Verification items for this drawing (mm, ordinates from the low corner). A direction names the side the tool comes from. Coordinates: 2 decimals unless noted, no trailing zeros. Write each loop counter-clockwise with the first axis right and the second up, starting at its lowest first coordinate (ties: lowest second). Pieces come first, ordered by that corner, then holes. Notation, with made-up numbers: (53.25, 40) -> (76.25, 40) arc R25 cw to (76.25, 59) -> close; hole circle Ø7 at (-33, 4.25). An arc over 180 degrees is marked (long way). Answer as CSV lines item,"result".
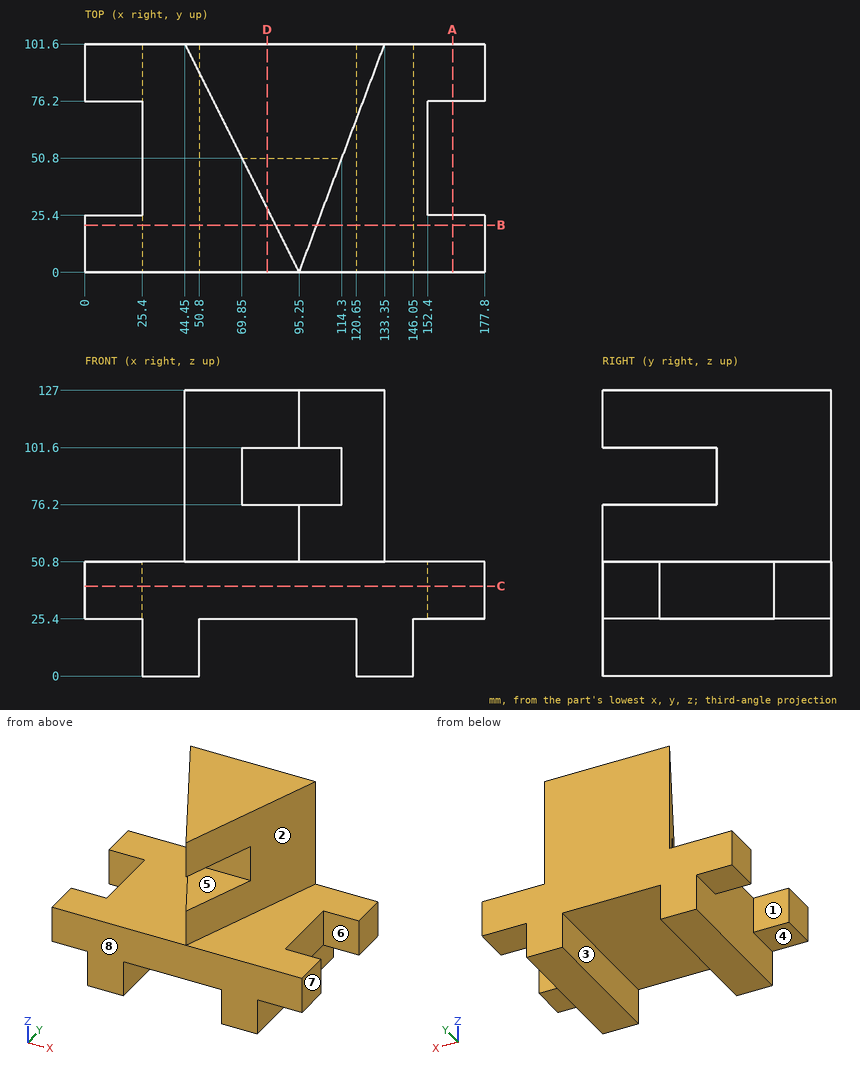
Item 1: Release check for a two-part mould opening along Y. For the marked faces 6, 7 and 8 record: +Y half, -Y half, draft (parallel to the pull), parting line (faces both ways), or undercut.
Responses:
face 6,"undercut"
face 7,"draft"
face 8,"-Y half"
Item 2: Cross-section at D-D, the plane x = 81. Record the cut outline in (y, z).
Responses:
outline,"(0, 25.4) -> (101.6, 25.4) -> (101.6, 127) -> (28.5, 127) -> (28.5, 101.6) -> (50.8, 101.6) -> (50.8, 76.2) -> (28.5, 76.2) -> (28.5, 50.8) -> (0, 50.8) -> close"
Item 3: Set-up check for the marked faces 1, 2, 3, 4 and 5: record each of +Z, -Z, +X, -X, +Y, -Y from which the full face is reachable in a straight line by a thin tool's end or side.
Responses:
face 1,"+Z, -Z, -X"
face 2,"+Z, +X, -Y"
face 3,"-Z, +Y, -Y"
face 4,"-Z, -X, +Y, -Y"
face 5,"+X, -X, -Y"
Item 4: Thickness scan on probe 1 along X at (y, z) = (32, 22); probe 2 along Z at (x, y) = (78, 89); probe 3 along Z at (x, y) = (152, 82.5). Record the ranges inside material, lowest first.
Responses:
probe 1,"x = 25.4 to 50.8, 120.65 to 146.05"
probe 2,"z = 25.4 to 127"
probe 3,"z = 25.4 to 50.8"
Item 5: Depth check by flat-ended pin: pin 1 Ø15 at (y, z) = (38, 22.5) entering from -X; pin 2 Ø4 at (x, y) = (91, 30.5) entering from -Z; pin 3 Ø1 at (x, y) = (53, 52.5) entering from +Z. Enter the tip coordinate at first touch or a pass-through.
Responses:
pin 1,"stops at x = 25.4"
pin 2,"stops at z = 25.4"
pin 3,"stops at z = 50.8"
Item 6: Cross-section at B-B, the plane y = 21. Record the cut outline in (x, z) (3 decimals).
Responses:
outline,"(0, 25.4) -> (25.4, 25.4) -> (25.4, 0) -> (50.8, 0) -> (50.8, 25.4) -> (120.65, 25.4) -> (120.65, 0) -> (146.05, 0) -> (146.05, 25.4) -> (177.8, 25.4) -> (177.8, 50.8) -> (103.125, 50.8) -> (103.125, 76.2) -> (84.75, 76.2) -> (84.75, 50.8) -> (0, 50.8) -> close; (84.75, 101.6) -> (103.125, 101.6) -> (103.125, 127) -> (84.75, 127) -> close"
Item 7: Cross-section at C-C, the plane z = 40. Record the cut outline in (x, y).
Responses:
outline,"(0, 0) -> (177.8, 0) -> (177.8, 25.4) -> (152.4, 25.4) -> (152.4, 76.2) -> (177.8, 76.2) -> (177.8, 101.6) -> (0, 101.6) -> (0, 76.2) -> (25.4, 76.2) -> (25.4, 25.4) -> (0, 25.4) -> close"
Item 8: Cross-section at A-A, the plane x = 163.5. Record the cut outline in (y, z), plus the area to 3 significant figures.
Responses:
outline,"(0, 25.4) -> (25.4, 25.4) -> (25.4, 50.8) -> (0, 50.8) -> close; (76.2, 25.4) -> (101.6, 25.4) -> (101.6, 50.8) -> (76.2, 50.8) -> close"
area,"1,290 mm2"
